Geometry: final body of the model. Coordinates: model frame, mm. A direction names the side the tool comes from. Round coordinates to 2 decimals unless told otherwise and drop trailing zeros. Loops run counter-clockwise (first coordinate to the right, second up) from the corner with the lowest first, then second, coordinate; pieces in that order, holes last. Notation, with made-up numbers: (9.5, -10) - (27.5, -10) arc R21 cw to (27.5, 9) - close; hole circle Ø5 at (13.25, 83). An arc over 180 degrees is marked (long way). Return JSON: item names as keys, results as strings. Group by question number.
1. Section A-A on x = 27.5. Return loops of the section in (y, z) (3 decimals), and give its area (3 significant figures).
2. Section C-C on y = -2.75. Return loops of the section in (x, z) (3 decimals).
3. Draft query along Z for faces 6 (the face through (-28.169, -3, -57)), 7 (the face through (-1, -3, -76.2)), 8 (the face through (-48.031, -3, -74)). Return one class per face: +Z half, -Z half, draft (parallel to the pull), parting line (faces both ways), or undercut.
4. Section B-B on z = -57.15. Return loops of the section in (x, y), and give its area (3 significant figures).
5. Material intervals for probe 1 along X at (y, z) = (-1.5, -57.15); probe 2 along X at (y, z) = (-5.25, -66); probe 3 along Z at (x, y) = (-10, -3.75) (3 decimals), sorted ascending.
6. Set-up query: faces 1 (the face through (-46, -3, -42.621)), 2 (the face through (-44.348, -3, -42)), 3 (the face through (1, 0, -61)), 4 (the face through (-48.031, -3, -39)), 5 (the face through (9, -3, -53.975)). Return all of +Z, -Z, +X, -X, +Y, -Y with unobstructed straight access to the full face (end or side cutting, diameter ignored); none if empty.
7. First-contact query: pin 1 Ø1.5 at (y, z) = (-3, -56) entering from +X; pin 2 Ø3 at (x, z) = (19.5, -58) entering from -Y; pin 3 Ø1.9 at (y, z) = (-3.5, -44.5) entering from -X. Flat tips, straight axial feed; report the tip coordinate or a pass-through.
from build123d import *

# Parameters (mm, degrees)
SKETCH1_R               = 1.8288
BOSS_EXTRUDE1_DEPTH     = 6.35
SKETCH2_W               = 96.0628
SKETCH2_H               = 111.337442597
CUT_EXTRUDE1_DEPTH      = 1
CUT_EXTRUDE1_DEPTH_BACK = 7.35


with BuildPart() as part:
    # Sketch1 → Boss-Extrude1 (new body)
    with BuildSketch(Plane(origin=(0, 0, 0), x_dir=(1, 0, 0), z_dir=(0, 1, 0))):
        Polygon((-48.0314, 76.2), (48.0314, 76.2), (48.0314, 60.325), (-28.1686, 60.325), (-28.1686, 53.975), (48.0314, 53.975), (48.0314, 22.225), (-28.1686, 22.225), (-28.1686, 15.875), (48.0314, 15.875), (48.0314, -15.875), (-28.1686, -15.875), (-28.1686, -22.225), (48.0314, -22.225), (48.0314, -53.975), (-28.1686, -53.975), (-28.1686, -60.325), (48.0314, -60.325), (48.0314, -76.2), (-48.0314, -76.2), (-48.0314, -33.5788), (-44.3484, -33.5788), (-44.3484, -35.687), (-41.6814, -35.687), (-41.6814, -27.813), (-44.3484, -27.813), (-44.3484, -29.9212), (-48.0314, -29.9212), (-48.0314, 4.5212), (-44.3484, 4.5212), (-44.3484, 2.413), (-41.6814, 2.413), (-41.6814, 10.287), (-44.3484, 10.287), (-44.3484, 8.1788), (-48.0314, 8.1788), (-48.0314, 42.6212), (-44.3484, 42.6212), (-44.3484, 40.513), (-41.6814, 40.513), (-41.6814, 48.387), (-44.3484, 48.387), (-44.3484, 46.2788), (-48.0314, 46.2788), (-48.0314, 68.0212), (-44.3484, 68.0212), (-44.3484, 65.913), (-41.6814, 65.913), (-41.6814, 73.787), (-44.3484, 73.787), (-44.3484, 71.6788), (-48.0314, 71.6788), align=None)
        with Locations((-38.1, 57.15)):
            Circle(SKETCH1_R, mode=Mode.SUBTRACT)
        with Locations((-38.1, 31.75)):
            Circle(SKETCH1_R, mode=Mode.SUBTRACT)
        with Locations((-38.1, 6.35)):
            Circle(SKETCH1_R, mode=Mode.SUBTRACT)
        with Locations((-38.1, -19.05)):
            Circle(SKETCH1_R, mode=Mode.SUBTRACT)
    extrude(amount=-BOSS_EXTRUDE1_DEPTH)

    # Sketch2 → Cut-Extrude1 (cut, two sides)
    with BuildSketch(Plane(origin=(0, 0, 0), x_dir=(1, 0, 0), z_dir=(0, 1, 0))) as cut_extrude1_sk:
        with Locations((0, -20.531278701)):
            Rectangle(SKETCH2_W, SKETCH2_H)
    extrude(amount=CUT_EXTRUDE1_DEPTH, mode=Mode.SUBTRACT)
    extrude(cut_extrude1_sk.sketch, amount=-CUT_EXTRUDE1_DEPTH_BACK, mode=Mode.SUBTRACT)


solid = part.part
Taken from the geometry:
{
 "1": {"outline": "(-6.35, -76.2) - (0, -76.2) - (0, -60.325) - (-6.35, -60.325) - close; (-6.35, -53.975) - (0, -53.975) - (0, -35.137) - (-6.35, -35.137) - close", "area": "220 mm2"},
 "2": {"outline": "(-48.031, -76.2) - (48.031, -76.2) - (48.031, -60.325) - (-28.169, -60.325) - (-28.169, -53.975) - (48.031, -53.975) - (48.031, -35.137) - (-48.031, -35.137) - (-48.031, -42.621) - (-44.348, -42.621) - (-44.348, -40.513) - (-41.681, -40.513) - (-41.681, -48.387) - (-44.348, -48.387) - (-44.348, -46.279) - (-48.031, -46.279) - (-48.031, -68.021) - (-44.348, -68.021) - (-44.348, -65.913) - (-41.681, -65.913) - (-41.681, -73.787) - (-44.348, -73.787) - (-44.348, -71.679) - (-48.031, -71.679) - close; hole circle Ø3.658 at (-38.1, -57.15)"},
 "3": {"face 6": "undercut", "face 7": "-Z half", "face 8": "draft"},
 "4": {"outline": "(-48.03, -6.35) - (-39.93, -6.35) - (-39.93, 0) - (-48.03, 0) - close; (-36.27, -6.35) - (-28.17, -6.35) - (-28.17, 0) - (-36.27, 0) - close", "area": "103 mm2"},
 "5": {"probe 1": "-48.03 to -39.93, -36.27 to -28.17", "probe 2": "-48.03 to -44.35, -41.68 to 48.03", "probe 3": "-76.2 to -60.325, -53.975 to -35.137"},
 "6": {"face 1": "-X, +Y, -Y", "face 2": "+Y, -Y", "face 3": "+Z, -Z, +X, -X, +Y", "face 4": "+Z, -Z, -X, +Y, -Y", "face 5": "+X, +Y, -Y"},
 "7": {"pin 1": "x = -28.17", "pin 2": "through", "pin 3": "x = -41.68"}
}
